Input: part model. Units: mm. Frame: model coordinates. A direction names the side the tool comes from. Coordinates: 2 decimals unless noted, no trailing zeros. Loops run counter-clockwise (first coordinate to the right, second up) from the corner with the lowest first, then second, coordinate; pieces in that order, holes last. Notation, with made-up numbers: M 23,-12 L 42,-12 A28 cw 42,22 Z; hole C 28,73 d4. An arc over 180 degrees is marked long. Use a Markdown table: item, result. Add a question column.
1. Section C-C on z = 10. Output: boundary loops of the cut face in (x, y).
2. Draft query along Y for faces 1 (the flat face through (4.514, 14.031, 13.176)), 2 (the flat face through (-3, 17.232, 10)), 3 (the flat face through (-17.905, -8.986, 1.52)), 4 (the cylindrical face through (2, 12.3, 7.9)). Return one class per face: +Y half, -Y half, draft (parallel to the pull), parting line (faces both ways), or undercut.
3. Section D-D on y = 6.5. Output: boundary loops of the cut face in (x, z).
4. Pin query (flat end, axial travel): pin 1 (5 mm diameter, centred on y = 12.23, z = 10, fed in from +X); pin 2 (0.6 mm diameter, centred on y = -9, z = 15.5, fed in from +X); pin 3 (1.5 mm diameter, centred on y = -2, z = 7.5, fed in from +X); pin 4 (6 mm diameter, centred on x = -1, y = 1, fed in from +Z). Return the tip coordinate at first contact, or that it passes through.
5. Section A-A on z = 16. Output: boundary loops of the cut face in (x, y).
6. Set-up query: faces 5 (the flat face through (-13, -8, 10)), 6 (the flat face through (4.514, 14.082, 6.854)), 7 (the cylindrical face through (-4.99, 8.67, 9.21)), 8 (the flat face through (-0.5, 12.2, 7.6)), 9 (the flat face through (-15.095, -8.986, 6.48)). Return all of +Z, -Z, +X, -X, +Y, -Y with unobstructed straight access to the full face (end or side cutting, diameter ignored); none if empty.
7. Section B-B on x = 1. Output: boundary loops of the cut face in (y, z).
8. Line query: L1, parallel to Z at x = -16.5, y = -12.1; L2, parallel to Y at x = 2, z = 11.5; L3, parallel to X at y = 16.5, z = 7. Output: solid intervals per line, ascending. Write a range as [from, to].
```python
from build123d import *

# Parameters (mm, degrees)
BOSS_EXTRUDE1_DEPTH     = 20
SKETCH2_R               = 2.1
CUT_EXTRUDE1_DEPTH      = 15.5
CUT_EXTRUDE1_DEPTH_BACK = 18.739
SKETCH4_R               = 3.65
CUT_EXTRUDE2_DEPTH      = 15.5
CUT_EXTRUDE2_DEPTH_BACK = 2
CUT_EXTRUDE3_DEPTH      = 7.7390001
CUT_EXTRUDE3_DEPTH_BACK = 2
SKETCH6_R               = 1.65
CUT_EXTRUDE4_DEPTH      = 6
CUT_EXTRUDE5_DEPTH      = 2
FILLET1_R               = 12


with BuildPart() as part:
    # Sketch1 → Boss-Extrude1 (new body)
    with BuildSketch(Plane.XY):
        with BuildLine():
            Line((-0.5, 7.221711778), (-0.5, 17.231747474))
            Line((-0.5, 17.231747474), (-5.5, 17.231747474))
            Line((-5.5, 17.231747474), (-5.5, 10.933577685))
            ThreePointArc((-5.5, 10.933577685), (-12.004275475, 2.385475074), (-9.262457611, -8))
            Line((-9.262457611, -8), (-20, -8))
            Line((-20, -8), (-20, -13))
            Line((-20, -13), (12.239, -13))
            Line((12.239, -13), (12.239, 0))
            ThreePointArc((12.239, 0), (10.418915994, 6.421784059), (5.5, 10.933577685))
            Line((5.5, 10.933577685), (5.5, 17.231747474))
            Line((5.5, 17.231747474), (0.5, 17.231747474))
            Line((0.5, 17.231747474), (0.5, 7.221711778))
            ThreePointArc((0.5, 7.221711778), (0, -7.239), (-0.5, 7.221711778))
        make_face()
    extrude(amount=BOSS_EXTRUDE1_DEPTH)

    # Sketch2 → Cut-Extrude1 (cut, two sides)
    with BuildSketch(Plane.ZY.offset(5.5)) as cut_extrude1_sk:
        with Locations((10, 12.231747474)):
            Circle(SKETCH2_R)
    extrude(amount=CUT_EXTRUDE1_DEPTH, mode=Mode.SUBTRACT)
    extrude(cut_extrude1_sk.sketch, amount=-CUT_EXTRUDE1_DEPTH_BACK, mode=Mode.SUBTRACT)

    # Sketch4 → Cut-Extrude2 (cut, two sides)
    with BuildSketch(Plane.ZY.offset(5.5)) as cut_extrude2_sk:
        with Locations((10, 12.231747474)):
            Circle(SKETCH4_R)
    extrude(amount=CUT_EXTRUDE2_DEPTH, mode=Mode.SUBTRACT)
    extrude(cut_extrude2_sk.sketch, amount=-CUT_EXTRUDE2_DEPTH_BACK, mode=Mode.SUBTRACT)

    # Sketch5 → Cut-Extrude3 (cut, two sides)
    with BuildSketch(Plane(origin=(5.5, 0, 0), x_dir=(0, 0, -1), z_dir=(1, 0, 0))) as cut_extrude3_sk:
        Polygon((-12.107328483, 8.581747474), (-14.214656965, 12.231747474), (-12.107328483, 15.881747474), (-7.892671517, 15.881747474), (-5.785343035, 12.231747474), (-7.892671517, 8.581747474), align=None)
    extrude(amount=CUT_EXTRUDE3_DEPTH, mode=Mode.SUBTRACT)
    extrude(cut_extrude3_sk.sketch, amount=-CUT_EXTRUDE3_DEPTH_BACK, mode=Mode.SUBTRACT)

    # Sketch6 → Cut-Extrude4 (cut, through all)
    with BuildSketch(Plane(origin=(0, -8, 0), x_dir=(1, 0, 0), z_dir=(0, 1, 0))):
        with Locations((-16.5, -4)):
            Circle(SKETCH6_R)
        with Locations((-16.5, -16)):
            Circle(SKETCH6_R)
    extrude(amount=-CUT_EXTRUDE4_DEPTH, mode=Mode.SUBTRACT)

    # Sketch7 → Cut-Extrude5 (cut)
    with BuildSketch(Plane(origin=(0, -8, 0), x_dir=(1, 0, 0), z_dir=(0, 1, 0))):
        Polygon((-16.5, -7.290896534), (-13.65, -5.645448267), (-13.65, -2.354551733), (-16.5, -0.709103466), (-19.35, -2.354551733), (-19.35, -5.645448267), align=None)
        Polygon((-16.5, -12.709103466), (-19.35, -14.354551733), (-19.35, -17.645448267), (-16.5, -19.290896534), (-13.65, -17.645448267), (-13.65, -14.354551733), align=None)
    extrude(amount=-CUT_EXTRUDE5_DEPTH, mode=Mode.SUBTRACT)

    # Fillet1
    fillet1_edges = [part.edges().sort_by_distance(p)[0] for p in [
        (12.239, -13, 10),
    ]]
    fillet(fillet1_edges, radius=FILLET1_R)


solid = part.part
```
Answers below:
| question | item | result |
|---|---|---|
| 1 | outline | M -20,-13 L 0.24,-13 A12 ccw 12.24,-1 L 12.24,0 A12.24 ccw 8.73,8.58 L 3.5,8.58 L 3.5,10.13 L 0.5,10.13 L 0.5,7.22 A7.24 cw long -0.5,7.22 L -0.5,10.13 L -3.5,10.13 L -3.5,8.58 L -8.73,8.58 A12.24 ccw -9.26,-8 L -20,-8 Z; M -5.5,15.88 L -3.5,15.88 L -3.5,14.33 L -0.5,14.33 L -0.5,17.23 L -5.5,17.23 Z; M 0.5,14.33 L 3.5,14.33 L 3.5,15.88 L 5.5,15.88 L 5.5,17.23 L 0.5,17.23 Z |
| 2 | face 1 | undercut |
| 2 | face 2 | +Y half |
| 2 | face 3 | draft |
| 2 | face 4 | undercut |
| 3 | outline | M -10.37,0 L -3.19,0 L -3.19,20 L -10.37,20 Z; M 3.19,0 L 10.37,0 L 10.37,20 L 3.19,20 Z |
| 4 | pin 1 | stops at x = 3.5 |
| 4 | pin 2 | stops at x = 9.44 |
| 4 | pin 3 | stops at x = 12.24 |
| 4 | pin 4 | passes through |
| 5 | outline | M -20,-13 L -18.15,-13 L -18.15,-10 L -19.35,-10 L -19.35,-8 L -20,-8 Z; M -14.85,-13 L 0.24,-13 A12 ccw 12.24,-1 L 12.24,0 A12.24 ccw 5.5,10.93 L 5.5,17.23 L 0.5,17.23 L 0.5,7.22 A7.24 cw long -0.5,7.22 L -0.5,17.23 L -5.5,17.23 L -5.5,10.93 A12.24 ccw -9.26,-8 L -13.65,-8 L -13.65,-10 L -14.85,-10 Z |
| 6 | face 5 | +Z, -Z, -X |
| 6 | face 6 | +X |
| 6 | face 7 | -X |
| 6 | face 8 | +Z, -Z, +Y |
| 6 | face 9 | +Y |
| 7 | outline | M -12.98,0 L -7.17,0 L -7.17,20 L -12.98,20 Z; M 7.17,0 L 17.23,0 L 17.23,20 L 7.17,20 Z; hole C 12.23,10 d4.2 |
| 8 | L1 | z = [0, 2.35], [5.65, 14.35], [17.65, 20] |
| 8 | L2 | y = [-12.87, -6.96], [6.96, 10.76], [13.7, 17.23] |
| 8 | L3 | x = [-5.5, -0.5], [0.5, 5.5] |
